Source: CAD feature listing. Evaluate the final solid. Frame: model axes, mm. A direction names the side the tool comes from. Coordinates: 2 decimals unless noted, no trailing zeros. Order: outer loops, then holes, each group sorted by start corner. A loop starts at its lowest first (then second) coordinate and runs counter-clockwise, first axis right, second up.
Item 1: Section D-D on x = 58. Return the cut outline in (y, z).
Item 2: Section B-B on x = 38. Return the cut outline in (y, z).
Item 3: Section C-C on y = 5. Return the cut outline in (x, z).
Item 4: Ray query, line 1 (X direction, y = 5, z = 5); line 2 (Z direction, x = 34.5, y = 3.75); line 3 (X direction, y = 6, z = -36). Return the intervals inside material, ascending.
Item 5: Mould query, pull axis Z, two halves, no side actions, for faces 1 (the cylindrical face through (42.35, 0.724, 7.841)), 2 (the flat face through (16, 5, -43.271)), 3 (the flat face through (66.299, 2, -13)), 4 (the flat face through (33.3, 4, -12)). Classes: released by +Z, released by -Z, zero draft, split by the parting line, or undercut.
Item 6: Reachability of faces 5 (the flat face through (51.08, 4, -12)), 6 (the cylindrical face through (51.844, 0.724, -12.919)), 7 (the flat face through (16, 5, 17.639)) from +Z, -Z, +X, -X, +Y, -Y: full face, straight path, thin tool, end or side. Return the list, or none.
Item 7: Contact query for flat-ended pins moving along their axis: P1, Ø1.1, axis at y = 5.5, z = -5.5, coming from the +X side; P2, Ø1.9, axis at x = 41, y = 5.5, coming from the -Z side; P3, Ø0.8, axis at y = 5.5, z = -21, coming from the -X side. Output: stop coordinate, or through.
Item 8: Section A-A on z = -12. Return the cut outline in (x, y), then the cut area to 3 significant figures.
from build123d import *

# Parameters (mm, degrees)
SKETCH1_W           = 108.824103019
SKETCH1_H           = 66.04
BOSS_EXTRUDE1_DEPTH = 3.81
SKETCH5_W           = 93.0148
SKETCH5_H           = 60.9092
BOSS_EXTRUDE2_DEPTH = 2.54
FILLET1_R           = 2.54
SKETCH6_W           = 17.78
SKETCH6_H           = 39.37
CUT_EXTRUDE1_DEPTH  = 7.366
FILLET2_R           = 2.54


with BuildPart() as part:
    # Sketch1 → Boss-Extrude1 (new body)
    with BuildSketch(Plane(origin=(0, 0, 0), x_dir=(1, 0, 0), z_dir=(0, 1, 0))):
        with Locations((11.887002401, 13.227171797)):
            Rectangle(SKETCH1_W, SKETCH1_H)
    extrude(amount=BOSS_EXTRUDE1_DEPTH)

    # Sketch5 → Boss-Extrude2 (add)
    with BuildSketch(Plane(origin=(0, 3.81, 0), x_dir=(1, 0, 0), z_dir=(0, 1, 0))):
        with Locations((16.711473858, 12.815998883)):
            Rectangle(SKETCH5_W, SKETCH5_H)
    extrude(amount=BOSS_EXTRUDE2_DEPTH)

    # Fillet1
    fillet1_edges = [part.edges().sort_by_distance(p)[0] for p in [
        (11.887002402, 0, -46.247171797),
        (11.887002402, 0, 19.792828203),
    ]]
    fillet(fillet1_edges, radius=FILLET1_R)

    # Sketch6 → Cut-Extrude1 (cut)
    with BuildSketch(Plane(origin=(0, 6.35, 0), x_dir=(1, 0, 0), z_dir=(0, 1, 0))):
        with Locations((42.189853997, 12.607362778)):
            Rectangle(SKETCH6_W, SKETCH6_H)
    extrude(amount=-CUT_EXTRUDE1_DEPTH, mode=Mode.SUBTRACT)

    # Fillet2
    fillet2_edges = [part.edges().sort_by_distance(p)[0] for p in [
        (42.189853997, 0, 7.077637222),
        (33.299853997, 0, -12.607362778),
        (42.189853997, 0, -32.292362778),
        (51.079853997, 0, -12.607362778),
    ]]
    fillet(fillet2_edges, radius=FILLET2_R)


solid = part.part
Answer list:
1. outline: (0, -43.71) arc R2.54 ccw to (2.54, -46.25) - (3.81, -46.25) - (3.81, -43.27) - (6.35, -43.27) - (6.35, 17.64) - (3.81, 17.64) - (3.81, 19.79) - (2.54, 19.79) arc R2.54 ccw to (0, 17.25) - close
2. outline: (0, -43.71) arc R2.54 ccw to (2.54, -46.25) - (3.81, -46.25) - (3.81, -43.27) - (6.35, -43.27) - (6.35, -32.29) - (2.54, -32.29) arc R2.54 ccw to (0, -34.83) - close; (0, 9.62) arc R2.54 ccw to (2.54, 7.08) - (6.35, 7.08) - (6.35, 17.64) - (3.81, 17.64) - (3.81, 19.79) - (2.54, 19.79) arc R2.54 ccw to (0, 17.25) - close
3. outline: (-29.8, -43.27) - (63.22, -43.27) - (63.22, 17.64) - (-29.8, 17.64) - close; hole (33.3, -32.29) - (51.08, -32.29) - (51.08, 7.08) - (33.3, 7.08) - close
4. line 1: x = -29.8 to 33.3, 51.08 to 63.22
4. line 2: z = -46.25 to -32.29, 7.08 to 19.79
4. line 3: x = -29.8 to 63.22
5. face 1: undercut
5. face 2: released by -Z
5. face 3: zero draft
5. face 4: undercut
6. face 5: +Y, -Y
6. face 6: -Y
6. face 7: +Z, +X, -X, +Y
7. P1: stops at x = 63.22
7. P2: stops at z = -43.27
7. P3: stops at x = -29.8
8. outline: (-42.53, 0) - (30.76, 0) arc R2.54 ccw to (33.3, 2.54) - (33.3, 6.35) - (-29.8, 6.35) - (-29.8, 3.81) - (-42.53, 3.81) - close; (51.08, 2.54) arc R2.54 ccw to (53.62, 0) - (66.3, 0) - (66.3, 3.81) - (63.22, 3.81) - (63.22, 6.35) - (51.08, 6.35) - close
8. area: 535 mm2
